```python
from build123d import *

# Parameters (mm, degrees)
EXTRUDE_1_DEPTH          = 30
SKETCH_2_R               = 1
CUT_EXTRUDE_4_DEPTH      = 31
CUT_EXTRUDE_4_DEPTH_BACK = 30
SKETCH_3_W               = 20
SKETCH_3_H               = 26
CUT_EXTRUDE_5_DEPTH      = 30
CUT_EXTRUDE_5_DEPTH_BACK = 30


with BuildPart() as part:
    # 草圖1 → 填料-伸長1 (new body)
    with BuildSketch(Plane.XY):
        with BuildLine():
            Line((-35, 5), (35, 5))
            ThreePointArc((35, 5), (40, 0), (35, -5))
            Line((35, -5), (-35, -5))
            ThreePointArc((-35, -5), (-40, 0), (-35, 5))
        make_face()
    extrude(amount=EXTRUDE_1_DEPTH)

    # 草圖2 → 除料-伸長4 (cut, two sides)
    with BuildSketch(Plane.XY) as cut_extrude_4_sk:
        with Locations((-35, 0)):
            Circle(SKETCH_2_R)
        with Locations((35, 0)):
            Circle(SKETCH_2_R)
    extrude(amount=CUT_EXTRUDE_4_DEPTH, mode=Mode.SUBTRACT)
    extrude(cut_extrude_4_sk.sketch, amount=-CUT_EXTRUDE_4_DEPTH_BACK, mode=Mode.SUBTRACT)

    # 草圖3 → 除料-伸長5 (cut, two sides)
    with BuildSketch(Plane(origin=(0, 0, 0), x_dir=(1, 0, 0), z_dir=(0, 1, 0))) as cut_extrude_5_sk:
        with Locations((-30, -15)):
            Rectangle(SKETCH_3_W, SKETCH_3_H)
        with Locations((30, -15)):
            Rectangle(SKETCH_3_W, SKETCH_3_H)
    extrude(amount=CUT_EXTRUDE_5_DEPTH, mode=Mode.SUBTRACT)
    extrude(cut_extrude_5_sk.sketch, amount=-CUT_EXTRUDE_5_DEPTH_BACK, mode=Mode.SUBTRACT)


solid = part.part
```
Could you check a few things on this model? Use its own coordinates, in mm. A direction names the side the tool comes from. Coordinates: 2 decimals unless noted, no trailing zeros. Write each loop counter-clockwise with the first axis right and the second up, starting at its lowest first coordinate (ties: lowest second). Pieces come first, ordered by that corner, then holes. Notation, with made-up numbers: (-28.75, 79) -> (-13.75, 79) arc R27 cw to (-13.75, 117) -> close; hole circle Ø6 at (88.25, -3.5). An arc over 180 degrees is marked (long way). Write item = value, one per line. Start each with the question number.
(1) I want a section at C-C (y = -4). Please give me the cut outline in (x, z), plus the area to 3 significant figures.
(2) Which directions (+Z, -Z, +X, -X, +Y, -Y) give clear straight access to the entire face, cutting with the end or side of a thin tool? Please do faces 4 (the face through (30, 0, 2)), 5 (the face through (-30, 0, 28)), 6 (the face through (40, 0, 29)).
(3) I want a section at B-B (y = 0). Please give me the cut outline in (x, z).
(4) We'd pull the mould along X, two halves only. Please class faces 1 (the face through (1, 0, 30)), 2 (the face through (-34, 0, 29)), 3 (the face through (-40, 0, 29)): released by +X, released by -X, zero draft, split by the parting line, or undercut.
(5) I want a section at D-D (z = 17.5). Please give me the cut outline in (x, y).
(6) I want a section at A-A (x = 30). Please give me the cut outline in (y, z), plus the area to 3 significant figures.
(7) Will these pins go through, and if not, where does the flat tip stop? pin 1 (12 mm diameter, centred on x = -31.5, z = 23.5, fed in from -Y); pin 2 (3 mm diameter, centred on y = 1, z = 11.5, fed in from +X); pin 3 (1.8 mm diameter, centred on x = -35, y = 0, fed in from -Z); pin 4 (3 mm diameter, centred on y = 4, z = 27, fed in from -X).
(8) I need wall thicknesses on line 1 (X direction, y = 0, z = 0.55); line 2 (Y direction, x = -35, z = 0.95); line 3 (Z direction, x = -30.5, y = -2). Which ranges of each line are inside material? Lowest first, please. Write a range as [from, to].
Result set:
q1.outline = (-38, 0) -> (38, 0) -> (38, 2) -> (20, 2) -> (20, 28) -> (38, 28) -> (38, 30) -> (-38, 30) -> (-38, 28) -> (-20, 28) -> (-20, 2) -> (-38, 2) -> close
q1.area = 1,340 mm2
q2.face_4 = +X, +Y, -Y
q2.face_5 = -X, +Y, -Y
q2.face_6 = +Z, -Z, +X
q3.outline = (-40, 0) -> (-36, 0) -> (-36, 2) -> (-40, 2) -> close; (-40, 28) -> (-36, 28) -> (-36, 30) -> (-40, 30) -> close; (-34, 0) -> (34, 0) -> (34, 2) -> (20, 2) -> (20, 28) -> (34, 28) -> (34, 30) -> (-34, 30) -> (-34, 28) -> (-20, 28) -> (-20, 2) -> (-34, 2) -> close; (36, 0) -> (40, 0) -> (40, 2) -> (36, 2) -> close; (36, 28) -> (40, 28) -> (40, 30) -> (36, 30) -> close
q4.face_1 = zero draft
q4.face_2 = undercut
q4.face_3 = released by -X
q5.outline = (-20, -5) -> (20, -5) -> (20, 5) -> (-20, 5) -> close
q6.outline = (-5, 0) -> (5, 0) -> (5, 2) -> (-5, 2) -> close; (-5, 28) -> (5, 28) -> (5, 30) -> (-5, 30) -> close
q6.area = 40.0 mm2
q7.pin_1 = -5
q7.pin_2 = 20
q7.pin_3 = through
q7.pin_4 = -39.09
q8.line_1 = [-40, -36], [-34, 34], [36, 40]
q8.line_2 = [-5, -1], [1, 5]
q8.line_3 = [0, 2], [28, 30]
